Read the model definition and answer for the solid it produces. Units are mm, in the model's axes. Face numbers are marked on the shaded views. A direction names the side the tool comes from. Round coordinates to 2 decimals unless told otherwise and drop trailing zeros. Loops run counter-clockwise (first coordinate to the right, second up) from the corner with the lowest first, then second, coordinate; pieces in that order, holes last. Notation, with made-up numbers: M -9.75,47 L 23.25,47 A22 cw 23.25,65 Z; hole C 32,-27.5 d1. An arc over 180 degrees is marked long. Write each question's results on one line, items separated by ' | '.
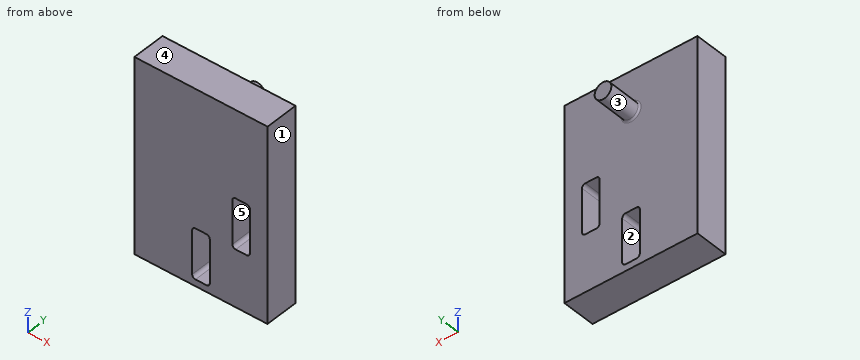
from build123d import *

# Parameters (mm, degrees)
BOSS_EXTRUDE1_DEPTH  = 10
FILLET2_R            = 1
FILLET2_OF_MIRROR1_R = 1
CUT_EXTRUDE1_DEPTH   = 81.635062113
FILLET3_R            = 1
SKETCH5_R            = 2.5
BOSS_EXTRUDE2_DEPTH  = 10
FILLET1_R            = 0.5
SKETCH6_W            = 39.78759817
SKETCH6_H            = 34
CUT_EXTRUDE2_DEPTH   = 10


with BuildPart() as part:
    # Sketch2 → Boss-Extrude1 (new body)
    with BuildSketch(Plane(origin=(0, 0, 0), x_dir=(1, 0, 0), z_dir=(0, 1, 0))):
        Polygon((-19.893799085, 77.5), (0, 77.5), (0, 75.5), (-2.625, 75.5), (-2.625, 73), (-2.625, 63), (-2.625, 60.5), (0, 60.5), (0, 60.375), (0, 2.5), (-2.625, 2.5), (-2.625, 0), (-2.625, -10), (-2.625, -12.5), (0, -12.5), (0, -14.5), (-19.893799085, -14.5), align=None)
    boss_extrude1 = extrude(amount=BOSS_EXTRUDE1_DEPTH)

    # Fillet2
    fillet2_edges = [part.edges().sort_by_distance(p)[0] for p in [
        (-2.625, 5, 12.5),
        (-2.625, 5, -2.5),
        (-2.625, 5, -60.5),
        (-2.625, 5, -75.5),
    ]]
    fillet(fillet2_edges, radius=FILLET2_R)

    # Mirror1: Boss-Extrude1 across Right Plane
    add(boss_extrude1.mirror(Plane(origin=(0, 0, 0), x_dir=(0, 0, -1), z_dir=(1, 0, 0))))

    # Fillet2 of Mirror1
    fillet2_of_mirror1_edges = [part.edges().sort_by_distance(p)[0] for p in [
        (2.625, 5, 12.5),
        (2.625, 5, -2.5),
        (2.625, 5, -60.5),
        (2.625, 5, -75.5),
    ]]
    fillet(fillet2_of_mirror1_edges, radius=FILLET2_OF_MIRROR1_R)

    # Sketch4 → Cut-Extrude1 (cut, through all)
    with BuildSketch(Plane(origin=(0, 0, 0), x_dir=(1, 0, 0), z_dir=(0, 1, 0))):
        Polygon((-14.625, 15), (-14.625, 5), (-14.625, 2.5), (-12, 2.5), (-9.375, 2.5), (-9.375, 5), (-9.375, 15), (-9.375, 17.5), (-12, 17.5), (-14.625, 17.5), align=None)
        Polygon((9.375, 58), (9.375, 48), (9.375, 45.5), (12, 45.5), (14.625, 45.5), (14.625, 48), (14.625, 58), (14.625, 60.5), (12, 60.5), (9.375, 60.5), align=None)
    extrude(amount=CUT_EXTRUDE1_DEPTH, mode=Mode.SUBTRACT)

    # Fillet3
    fillet3_edges = [part.edges().sort_by_distance(p)[0] for p in [
        (-14.625, 5, -17.5),
        (-14.625, 5, -2.5),
        (-9.375, 5, -2.5),
        (-9.375, 5, -17.5),
        (14.625, 5, -60.5),
        (9.375, 5, -60.5),
        (9.375, 5, -45.5),
        (14.625, 5, -45.5),
    ]]
    fillet(fillet3_edges, radius=FILLET3_R)

    # Sketch5 → Boss-Extrude2 (add)
    with BuildSketch(Plane(origin=(0, 10, 0), x_dir=(1, 0, 0), z_dir=(0, 1, 0))):
        with Locations(Location((0, 31.5, 0), (0, 0, 90))):
            Circle(SKETCH5_R)
    extrude(amount=BOSS_EXTRUDE2_DEPTH)

    # Fillet1
    fillet1_edges = [part.edges().sort_by_distance(p)[0] for p in [
        (0, 10, -29),
    ]]
    fillet(fillet1_edges, radius=FILLET1_R)

    # Sketch6 → Cut-Extrude2 (cut)
    with BuildSketch(Plane(origin=(0, 10, 0), x_dir=(1, 0, 0), z_dir=(0, 1, 0))):
        with Locations((0, 2.5)):
            Rectangle(SKETCH6_W, SKETCH6_H)
    extrude(amount=-CUT_EXTRUDE2_DEPTH, mode=Mode.SUBTRACT)


solid = part.part
Item 1: The part is cut by section C-C (z = -64.5). Determine the outline of the cut face in (x, y) (3 decimals), plus the area to 3 significant figures.
Outcome:
outline: M -19.894,0 L -2.625,0 L -2.625,10 L -19.894,10 Z; M 2.625,0 L 19.894,0 L 19.894,10 L 2.625,10 Z | area: 345 mm2
Item 2: The mould has two halves that part along Z. Classify the marked faces 1, 2 and 3: pulls with the +Z half, pulls with the -Z half, needs draft (parallel to the pull), parting line crosses it, or undercut.
Outcome:
face 1: needs draft | face 2: undercut | face 3: parting line crosses it
Item 3: The part is cut by section B-B (y = 6). Determine the outline of the cut face in (x, z) (3 decimals), plus the area to 3 significant figures.
Outcome:
outline: M -19.894,-77.5 L 19.894,-77.5 L 19.894,-19.5 L -19.894,-19.5 Z; hole M -2.625,-74.5 A1 ccw -1.625,-75.5 L 1.625,-75.5 A1 ccw 2.625,-74.5 L 2.625,-61.5 A1 ccw 1.625,-60.5 L -1.625,-60.5 A1 ccw -2.625,-61.5 Z; hole M 9.375,-59.5 A1 ccw 10.375,-60.5 L 13.625,-60.5 A1 ccw 14.625,-59.5 L 14.625,-46.5 A1 ccw 13.625,-45.5 L 10.375,-45.5 A1 ccw 9.375,-46.5 Z | area: 2,150 mm2
Item 4: The part is cut by section D-D (x = 11.5). Determine the outline of the cut face in (y, z).
Outcome:
outline: M 0,-77.5 L 10,-77.5 L 10,-60.5 L 0,-60.5 Z; M 0,-45.5 L 10,-45.5 L 10,-19.5 L 0,-19.5 Z
Item 5: For the marked faces 4 and 5, determine the directions among +Z, -Z, +X, -X, +Y, -Y from which every point of the face is accessible in a straight line to the end or side of a thin tool.
Outcome:
face 4: +Z, +X, -X, +Y, -Y | face 5: +Y, -Y
Item 6: The part is cut by section A-A (x = 0). Determine the outline of the cut face in (y, z).
Outcome:
outline: M 0,-77.5 L 10,-77.5 L 10,-75.5 L 0,-75.5 Z; M 0,-60.5 L 10,-60.5 L 10,-34.5 A0.5 cw 10.5,-34 L 20,-34 L 20,-29 L 10.5,-29 A0.5 cw 10,-28.5 L 10,-19.5 L 0,-19.5 Z
Item 7: Straight lines are drawn through the part: line 1 (X direction, y = 1.5, z = -69) (3 decimals); line 2 (X direction, y = 8.75, z = -50) (3 decimals); line 3 (Y direction, x = -17, z = -33). For each, find the intervals that lie inside material, in ascending order.
Outcome:
line 1: x = -19.894 to -2.625, 2.625 to 19.894 | line 2: x = -19.894 to 9.375, 14.625 to 19.894 | line 3: y = 0 to 10
